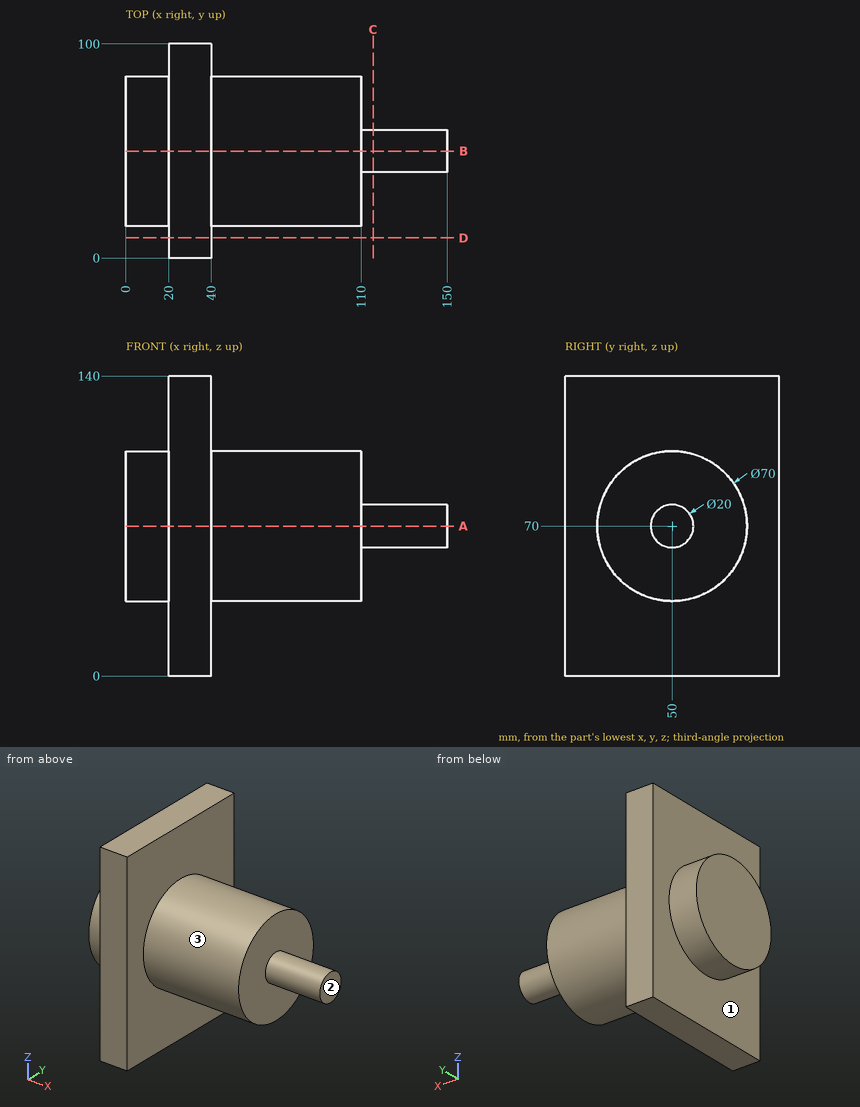
Print and shaded views of the part. All mm, measured from the part's lowest x, y and z. A direction names the side the tool comes from. Give positions to 0.01 mm unless a question says otherwise; leave off trailing zeros. Loops run counter-clockwise (first coordinate to the right, second up) from the corner with the lowest first, then second, coordinate; pieces in that order, holes last. Notation, with made-up numbers: (-28.75, 77.25) -> (27.25, 77.25) arc R16 ccw to (27.25, 96.25) -> close; hole circle Ø9 at (87, 16.5). An arc over 180 degrees is marked (long way). One line per question, with ' | ' between items. Start each with the question number.
1) Pin check, flat tips, straight feed: pin 1 (6 mm diameter, centred on x = 105.5, z = 93.5, fed in from -Y); pin 2 (3 mm diameter, centred on x = 99.5, y = 53, fed in from +Z); pin 3 (5 mm diameter, centred on x = 117, y = 57, fed in from +Z). Stop position of each tip, or through.
2) Cut at D-D (y = 9.5). Give the cut face in (x, z), plus the area to 3 significant figures.
3) 3-axis set-ups, long thin cutter, end or side, ignore diameter. For the marked faces 1, 2 and 3: which of +Z, -Z, +X, -X, +Y, -Y reach the whole face in a straight line?
4) Cut at B-B (y = 50). Give the cut face in (x, z).
5) Cut at C-C (x = 115.5). Give the cut face in (y, z), plus the area to 3 significant figures.
6) Cut at A-A (z = 70). Give the cut face in (x, y).
7) Probe L1, parallel to Y at x = 108, z = 52; L2, parallel to X at y = 16, z = 22; L3, parallel to X at y = 64, z = 70. List the from-to ranges inside material, lowest first.
Return value:
1) pin 1: y = 21.63 | pin 2: z = 104.97 | pin 3: z = 78.93
2) outline: (20, 0) -> (40, 0) -> (40, 140) -> (20, 140) -> close | area: 2,800 mm^2
3) face 1: -X | face 2: +Z, -Z, +X, +Y, -Y | face 3: +X
4) outline: (0, 35) -> (20, 35) -> (20, 0) -> (40, 0) -> (40, 35) -> (110, 35) -> (110, 60) -> (150, 60) -> (150, 80) -> (110, 80) -> (110, 105) -> (40, 105) -> (40, 140) -> (20, 140) -> (20, 105) -> (0, 105) -> close
5) outline: circle Ø20 at (50, 70) | area: 314 mm^2
6) outline: (0, 15) -> (20, 15) -> (20, 0) -> (40, 0) -> (40, 15) -> (110, 15) -> (110, 40) -> (150, 40) -> (150, 60) -> (110, 60) -> (110, 85) -> (40, 85) -> (40, 100) -> (20, 100) -> (20, 85) -> (0, 85) -> close
7) L1: 19.98 to 80.02 | L2: 20 to 40 | L3: 0 to 110
